Part model, mm, in its own coordinate system. Face numbers are marked on the shaded views. Round coordinates to 2 decimals unless told otherwise and drop trailing zeros. Write each loop counter-clockwise with the first axis right and the second up, starting at its lowest first coordinate (ties: lowest second). Pieces come first, ordered by that corner, then holes. Notation, with made-up numbers: (10, 65) -> (48, 65) arc R19 ccw to (48, 96) -> close; hole circle Ø9 at (53, 44). An arc over 180 degrees is marked (long way). Return JSON: item names as keys, results as strings. Group by question number.
(1) Mould opens along X. For the marked faces 1 and 2 say: +X half, -X half, draft (parallel to the pull), parting line (faces both ways), or undercut.
(2) Drill centre lines: L1, parallel to Y at x = 0.5, z = 0.5; L2, parallel to X at y = -10.5, z = 3; L3, parallel to Y at x = -14.5, z = 1. Where is each one in solid material? Low to high. Write a range as from..to.
(3) Saw through at B-B (y = 0). List the corners of the cut face in (x, z), plus the area to 3 significant figures.
(4) Saw through at A-A (z = 3.25). List the corners of the cut face in (x, y), plus the area to 3 significant figures.
(5) Drop flat-ended pins along their axis: pin 1 Ø3 at (x, z) = (-39.5, 3) entering from +Y; pin 2 Ø3 at (x, z) = (39, 2.5) entering from +Y; pin 3 Ø1.5 at (y, z) = (21, 2) entering from -X. Give the stop position or say it passes through.
from build123d import *

# Parameters (mm, degrees)
SKETCH_1_R               = 41
EXTRUDE_1_DEPTH          = 6
HOLE_WIZARD_M64_1_D      = 58
CHAMFER_1_SIZE           = 1
SKETCH_5_W               = 3
SKETCH_5_H               = 5
CUT_EXTRUDE_1_DEPTH      = 59.292366567
PATTERN_CIRCULAR_1_COUNT = 4


with BuildPart() as part:
    # 草图1 → 凸台-拉伸1 (new body)
    with BuildSketch(Plane.XY):
        Circle(SKETCH_1_R)
    extrude(amount=EXTRUDE_1_DEPTH)

    # M64 螺纹孔1 (through all)
    with Locations(Plane.XY.offset(6)):
        with Locations((0, 0)):
            Hole(HOLE_WIZARD_M64_1_D / 2)

    # 倒角1
    chamfer_1_edges = [part.edges().sort_by_distance(p)[0] for p in [
        (-41, 0, 0),
        (-41, 0, 6),
    ]]
    chamfer(chamfer_1_edges, length=CHAMFER_1_SIZE)

    # 草图5 → 切除-拉伸1 (cut, through all)
    with BuildSketch(Plane.XY.offset(6)):
        with Locations((39.5, 0)):
            Rectangle(SKETCH_5_W, SKETCH_5_H)
    cut_extrude_1 = extrude(amount=-CUT_EXTRUDE_1_DEPTH, mode=Mode.SUBTRACT)

    # 阵列(圆周)1: 切除-拉伸1 ×4 about axis
    pattern_circular_1_axis = Axis((0, 0, 0), (0, 0, 1))
    for i in range(1, PATTERN_CIRCULAR_1_COUNT):
        add(cut_extrude_1.rotate(pattern_circular_1_axis, i * 360 / PATTERN_CIRCULAR_1_COUNT), mode=Mode.SUBTRACT)


solid = part.part
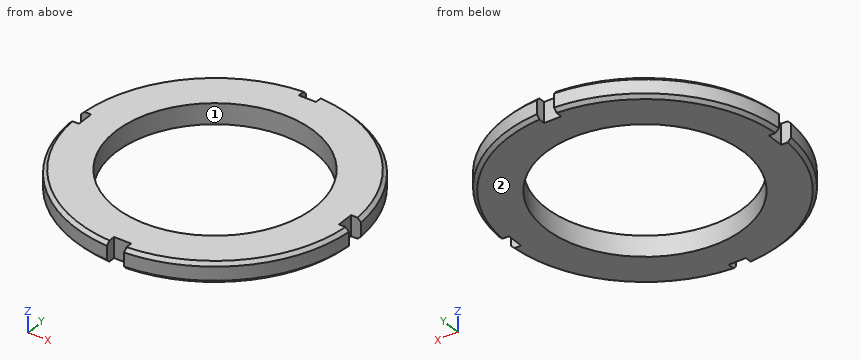
Computed values:
{
 "1": {"face 1": "undercut", "face 2": "draft"},
 "2": {"L1": "-38..-29, 29..38", "L2": "-39.63..-27.03, 27.03..39.63", "L3": "-38.35..-25.11, 25.11..38.35"},
 "3": {"outline": "(-38, 0) -> (-29, 0) -> (-29, 6) -> (-38, 6) -> close; (29, 0) -> (38, 0) -> (38, 6) -> (29, 6) -> close", "area": "108 mm2"},
 "4": {"outline": "(-40.92, -2.5) arc R41 ccw to (-2.5, -40.92) -> (-2.5, -38) -> (2.5, -38) -> (2.5, -40.92) arc R41 ccw to (40.92, -2.5) -> (38, -2.5) -> (38, 2.5) -> (40.92, 2.5) arc R41 ccw to (2.5, 40.92) -> (2.5, 38) -> (-2.5, 38) -> (-2.5, 40.92) arc R41 ccw to (-40.92, 2.5) -> (-38, 2.5) -> (-38, -2.5) -> close; hole circle Ø58 at (0, 0)", "area": "2,580 mm2"},
 "5": {"pin 1": "y = 15.39", "pin 2": "y = 16.58", "pin 3": "x = -35.65"}
}
